CAD build for the part. Positions are in the model's coordinates, mm. A direction names the side the tool comes from. Give positions to 0.01 mm unless a question says otherwise; leave off trailing zeros. Order: outer loops, then holes, each group sorted by start corner. A loop starts at its lowest first (then second) coordinate and runs counter-clockwise, first axis right, second up.
Item 1: Wall check: L1, parallel to Y at x = 0, z = 24; L2, parallel to Y at x = 1.5, z = 15.5; L3, parallel to Y at x = 13.5, z = 11. Give the ranges that are in metal, low to high.
Item 2: Band-saw the part on C-C on x = 0. Give the cut face in (y, z).
Item 3: Band-saw the part on A-A on y = 0. Give the cut face in (x, z), plus the area to 3 significant figures.
Item 4: Flat gauge pins, fed straight in: P1, Ø4, axis at x = 5, z = 16.5, coming from the -Y side; P2, Ø2, axis at y = -11.5, z = 7.5, coming from the +X side; P3, Ø5.5, axis at x = 4, z = 15, coming from the -Y side. Where does each tip first touch, or does it go through?
Item 5: Which spindle directions (+Z, -Z, +X, -X, +Y, -Y) get a long thin tool onto all of the face, cutting with end or side? Do faces 1 (the flat face through (9.25, 0, 15)), 2 (the cylindrical face through (-13.887, -10.648, 9.86)). Say none if no direction does.
Item 6: Band-saw the part on B-B on z = 8.75. Give the cut face in (x, y).
```python
from build123d import *

# Parameters (mm, degrees)
F0_R     = 17.5
F1_DEPTH = 25
F2_R     = 5
F3_W     = 18.5
F3_H     = 1.7
F4_DEPTH = 20


with BuildPart() as f1:
    # F0 (on Top) → F1 (new body)
    with BuildSketch(Plane.XY):
        Circle(F0_R)
    extrude(amount=F1_DEPTH)

    # F2
    f2_edges = [f1.edges().sort_by_distance(p)[0] for p in [
        (-17.5, 0, 25),
    ]]
    fillet(f2_edges, radius=F2_R)

    # F3 (on face) → F4 (cut)
    with BuildSketch(Plane.XY.offset(25)):
        Rectangle(F3_W, F3_H)
    extrude(amount=-F4_DEPTH, mode=Mode.SUBTRACT)


solid = f1.part
```
The answers:
1. L1: y = -15.5 to -0.85, 0.85 to 15.5
1. L2: y = -17.44 to -0.85, 0.85 to 17.44
1. L3: y = -11.14 to 11.14
2. outline: (-17.5, 0) - (17.5, 0) - (17.5, 20) arc R5 ccw to (12.5, 25) - (0.85, 25) - (0.85, 5) - (-0.85, 5) - (-0.85, 25) - (-12.5, 25) arc R5 ccw to (-17.5, 20) - close
3. outline: (-17.5, 0) - (17.5, 0) - (17.5, 20) arc R5 ccw to (12.5, 25) - (9.25, 25) - (9.25, 5) - (-9.25, 5) - (-9.25, 25) - (-12.5, 25) arc R5 ccw to (-17.5, 20) - close
3. area: 494 mm2
4. P1: stops at y = -17.24
4. P2: stops at x = 14
4. P3: stops at y = -17.46
5. face 1: +Z
5. face 2: +Z, -Z
6. outline: circle Ø35 at (0, 0); hole (-9.25, -0.85) - (9.25, -0.85) - (9.25, 0.85) - (-9.25, 0.85) - close
